Design review of the part built by this model. Coordinates are the model's own, in mm. A direction names the side the tool comes from. Round coordinates to 2 decimals unless told otherwise and drop trailing zeros. Write each loop counter-clockwise with the first axis right and the second up, starting at its lowest first coordinate (ties: lowest second). Pieces come first, ordered by that corner, then holes.
from build123d import *

# Parameters (mm, degrees)
SKETCH_1_R      = 1.75
EXTRUDE_1_DEPTH = 3
SKETCH_2_R      = 1.75
EXTRUDE_2_DEPTH = 3
EXTRUDE_3_DEPTH = 7.5
SKETCH_4_R      = 6
EXTRUDE_4_DEPTH = 4
FILLET_1_R      = 2
CHAMFER_1_SIZE  = 2


with BuildPart() as part:
    # 草图1 → 凸台-拉伸1 (new body)
    with BuildSketch(Plane.XY):
        with BuildLine():
            Line((8.162825685, 0), (-8.162825685, 0))
            Line((-8.162825685, 0), (-16.496696216, 11.833026185))
            ThreePointArc((-16.496696216, 11.833026185), (-15.768394863, 19.006145299), (-8.564177238, 19.294778452))
            ThreePointArc((-8.564177238, 19.294778452), (0, 16.290627288), (8.564177238, 19.294778452))
            ThreePointArc((8.564177238, 19.294778452), (15.768394863, 19.006145299), (16.496696216, 11.833026185))
            Line((16.496696216, 11.833026185), (8.162825685, 0))
        make_face()
        with Locations((-12, 15)):
            Circle(SKETCH_1_R, mode=Mode.SUBTRACT)
        with Locations(Location((12, 15, 0), (0, 0, 180))):
            Circle(SKETCH_1_R, mode=Mode.SUBTRACT)
    extrude(amount=EXTRUDE_1_DEPTH)

    # 草图2 → 凸台-拉伸2 (add)
    with BuildSketch(Plane.XZ):
        with BuildLine():
            Line((8.162825685, 0), (-8.162825685, 0))
            Line((-8.162825685, 0), (-16.708682104, 14.157762704))
            ThreePointArc((-16.708682104, 14.157762704), (-15.476402024, 21.261998237), (-8.269459435, 21.041418945))
            ThreePointArc((-8.269459435, 21.041418945), (0, 17.808193987), (8.269459435, 21.041418945))
            ThreePointArc((8.269459435, 21.041418945), (15.476402024, 21.261998237), (16.708682104, 14.157762704))
            Line((16.708682104, 14.157762704), (8.162825685, 0))
        make_face()
        with Locations(Location((-12, 17, 0), (0, 0, 270))):
            Circle(SKETCH_2_R, mode=Mode.SUBTRACT)
        with Locations(Location((12, 17, 0), (0, 0, 90))):
            Circle(SKETCH_2_R, mode=Mode.SUBTRACT)
    extrude(amount=-EXTRUDE_2_DEPTH)

    # 草图3 → 凸台-拉伸3 (add, symmetric)
    with BuildSketch(Plane(origin=(0, 0, 0), x_dir=(0, 0, -1), z_dir=(1, 0, 0))):
        Polygon((-3, 3), (-17, 3), (-3, 14.571172971), align=None)
    extrude(amount=EXTRUDE_3_DEPTH, both=True)

    # 草图4 → 凸台-拉伸4 (add)
    with BuildSketch(Plane(origin=(0, 10.130402441, 8.372902779), x_dir=(1, 0, 0), z_dir=(0, 0.7708007256408878, 0.6370763230190564))):
        with Locations(Location((0, 0, 0), (0, 0, 90))):
            Circle(SKETCH_4_R)
        Polygon((0, 2), (-1.732050808, 1), (-1.732050808, -1), (0, -2), (1.732050808, -1), (1.732050808, 1), align=None, mode=Mode.SUBTRACT)
    extrude(amount=EXTRUDE_4_DEPTH)

    # 圆角1
    fillet_1_edges = [part.edges().sort_by_distance(p)[0] for p in [
        (0, 9.391147406, 15.546012425),
    ]]
    fillet(fillet_1_edges, radius=FILLET_1_R)

    # 倒角1
    chamfer_1_edges = [part.edges().sort_by_distance(p)[0] for p in [
        (-13.75, 15, 3),
        (13.75, 15, 3),
        (12, 3, 15.25),
        (-12, 3, 18.75),
    ]]
    chamfer(chamfer_1_edges, length=CHAMFER_1_SIZE)


solid = part.part
1) For faces 5 (the face through (7.5, 6, 7)), 6 (the face through (-12.27, 5.83, 1.48)), 7 (the face through (15.69, 19.08, 1.48)), 8 (the face through (0.88, 12.6, 8.48)), 9 (the face through (15.39, 1.48, 21.33)), list the 3-axis set-ups (+Z, -Z, +X, -X, +Y, -Y) from which the entire face can be reached by the end or side of a thin tool; tool diameter is ignored.
2) Add section C-C on y = 4. State the section outline as (x, z) points, and give its area (3 significant figures).
3) Add section B-B on z = 18.25. Count the separate pieces of the cut face and the enclosed holes in it, and give its area (3 significant figures).
4) For P1, Ø6, axis at y = 8, z = 13, coming from the -X side; P2, Ø9, axis at x = 4, y = 15, coming from the +Z side; P3, Ø3.5, axis at y = 12, z = 9.5, coming from the -X side, all flat-tipped, find the tip position at first contact; note any pin that passes through.
5) The part is to be moulded in two halves that separate along X. For faces 1 (the face through (0.833, 14.311, 9.594)), 2 (the face through (-7.5, 6, 7)), 3 (the face through (-15.85, 18.93, 1.48)), 4 (the face through (-0.854, 12.61, 8.468)), say which applies: pulls with the +X half, pulls with the -X half, needs draft (parallel to the pull), parting line crosses it, or undercut.
6) For line 1 along X through (y, z) = (0.45, 17); line 2 along X through (y, z) = (1.75, 17); line 3 along Y through (x, z) = (-9, 6.5), list the stretches that pass through material, from the lowest coordinate up.
7) Add section A-A on x = -12. State the section outline as (y, z) points, and give its area (3 significant figures).
Computed:
1. face 5: +Z, +X, +Y
1. face 6: -Z, -X, -Y
1. face 7: +Z, -Z
1. face 8: none
1. face 9: +Y, -Y
2. outline: (-10.98, 0) - (10.98, 0) - (10.98, 3) - (7.5, 3) - (7.5, 15.79) - (-7.5, 15.79) - (-7.5, 3) - (-10.98, 3) - close
2. area: 258 mm2
3. separate pieces: 4
3. enclosed holes: 0
3. area: 60.3 mm2
4. P1: stops at x = -7.5
4. P2: stops at z = 13.79
4. P3: stops at x = -6
5. face 1: needs draft
5. face 2: pulls with the -X half
5. face 3: undercut
5. face 4: undercut
6. line 1: x = -17.5 to -13.75, -10.25 to 10.25, 13.75 to 17.5
6. line 2: x = -17.5 to -14.5, -9.5 to 9.5, 14.5 to 17.5
6. line 3: y = 0 to 3
7. outline: (0, 6.36) - (3, 6.36) - (3, 13.25) - (1, 15.25) - (0, 15.25) - close; (0, 18.75) - (1, 18.75) - (3, 20.75) - (3, 22.5) - (0, 22.5) - close; (5.45, 0) - (13.25, 0) - (13.25, 1) - (11.25, 3) - (5.45, 3) - close; (16.75, 0) - (20.5, 0) - (20.5, 3) - (18.75, 3) - (16.75, 1) - close
7. area: 64.6 mm2
